Geometry: see drawing. Coordinates: mm, zero at the bounding-box minimum. Give positions to 0.01 mm unless a question says otherwise; leave off trailing zeros. Write each loop counter-clockwise with the first axis right and the second up, starting at its lowest first coordinate (ties: lowest second). Pieces come first, ordered by that corner, then holes. Notation, with made-up numbers: (3.5, 16.5) - (52.5, 16.5) arc R16 cw to (52.5, 41.5) - close; hole circle Ø5 at (84, 69.25). An arc over 180 degrees is marked (long way). Use a Markdown table: item, result. Add a question column.
1. Section query A-A, the plane z = 6. Return loops of the section in (x, y), plus the area to 3 significant figures.
2. Section query B-B, the plane x = 9.25. Return loops of the section in (y, z).
3. Mould query, pull axis X, two halves, no side actions, for the marked faces 1, 2, 3 and 4. Classes: released by +X, released by -X, zero draft, split by the parting line, or undercut.
4. Pin query (flat end, axial travel): pin 1 (4 mm diameter, centred on x = 10.34, z = 6, fed in from -Y). Return the tip coordinate at first contact, or that it passes through.
5. Section query D-D, the plane x = 7.5. Return loops of the section in (y, z), plus the area to 3 significant figures.
6. Material intervals for probe 1 along Z at (x, y) = (10.25, 2); probe 2 along Z at (x, y) = (9.25, 2.5); probe 3 along X at (y, z) = (9.75, 6.5), sorted ascending.
7. Section query C-C, the plane y = 4.75. Return loops of the section in (x, z).
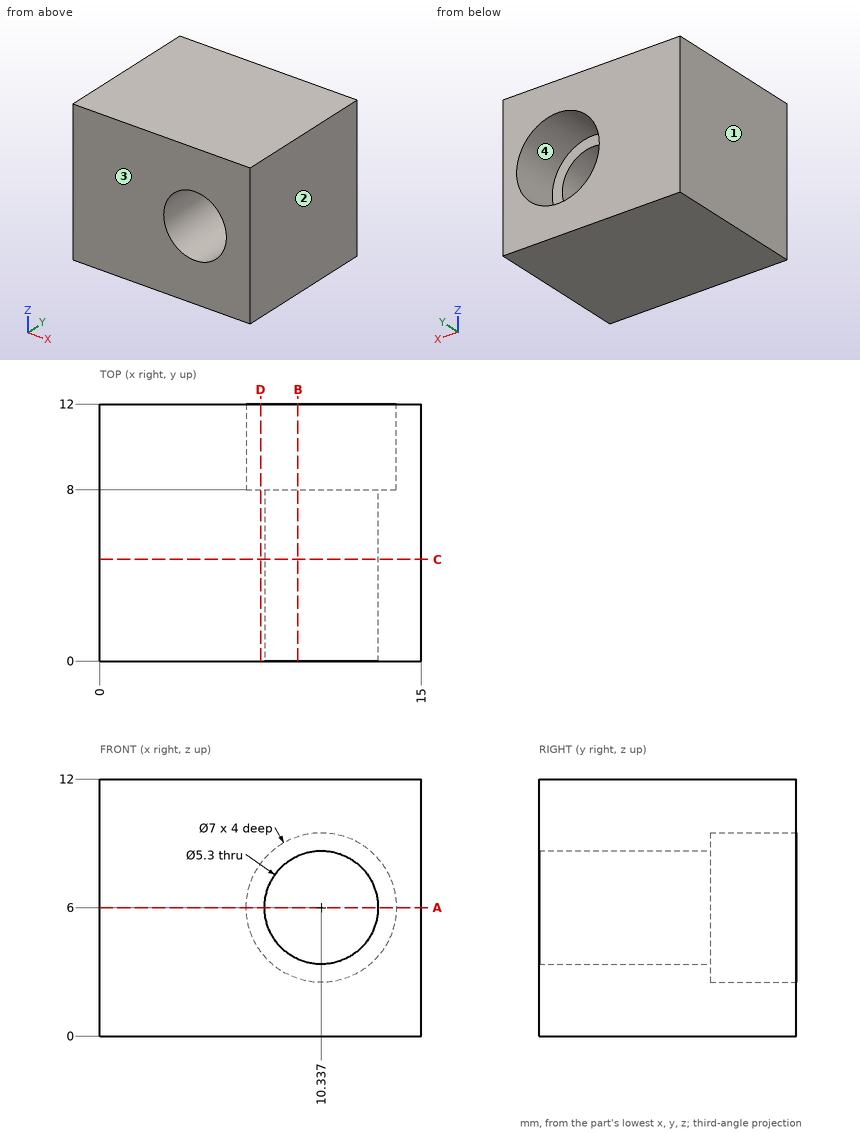
Result sheet:
| question | item | result |
|---|---|---|
| 1 | outline | (0, 0) - (7.69, 0) - (7.69, 8) - (6.84, 8) - (6.84, 12) - (0, 12) - close; (12.99, 0) - (15, 0) - (15, 12) - (13.84, 12) - (13.84, 8) - (12.99, 8) - close |
| 1 | area | 110 mm² |
| 2 | outline | (0, 0) - (12, 0) - (12, 2.67) - (8, 2.67) - (8, 3.58) - (0, 3.58) - close; (0, 8.42) - (8, 8.42) - (8, 9.33) - (12, 9.33) - (12, 12) - (0, 12) - close |
| 3 | face 1 | released by -X |
| 3 | face 2 | released by +X |
| 3 | face 3 | zero draft |
| 3 | face 4 | undercut |
| 4 | pin 1 | passes through |
| 5 | outline | (0, 0) - (12, 0) - (12, 3.95) - (8, 3.95) - (8, 8.05) - (12, 8.05) - (12, 12) - (0, 12) - close |
| 5 | area | 128 mm² |
| 6 | probe 1 | z = 0 to 3.35, 8.65 to 12 |
| 6 | probe 2 | z = 0 to 3.58, 8.42 to 12 |
| 6 | probe 3 | x = 0 to 6.87, 13.8 to 15 |
| 7 | outline | (0, 0) - (15, 0) - (15, 12) - (0, 12) - close; hole circle Ø5.3 at (10.34, 6) |
